Work out the finished part from the listing and answer in its coordinate system (mm). A direction names the side the tool comes from. Round coordinates to 2 decimals unless told otherwise and drop trailing zeros. Order: outer loops, then holes, each group sorted by start corner. A loop starts at its lowest first (then second) coordinate and runs counter-clockwise, first axis right, second up. Notation, with made-up numbers: (-15, 89.5) - (-8, 89.5) arc R34 cw to (-8, 125.5) - close; hole circle Ø4 at (-11, 54). An arc over 180 degrees is marked (long way). Answer in a Markdown table with one row per item.
from build123d import *

# Parameters (mm, degrees)
SCHIZZO1_R                   = 7.5
SCHIZZO1_R_2                 = 2
ESTRUSIONE_ESTRUSIONE1_DEPTH = 4


with BuildPart() as part:
    # Schizzo1 → Estrusione-Estrusione1 (new body)
    with BuildSketch(Plane.XY):
        Polygon((0, 90), (0, 0), (35, 0), (35, -4), (45, -4), (45, 0), (135, 0), (135, -4), (145, -4), (145, 0), (235, 0), (235, -4), (245, -4), (245, 0), (335, 0), (335, -4), (345, -4), (345, 0), (435, 0), (435, -4), (445, -4), (445, 0), (490, 0), (490, 90), (445, 90), (445, 94), (435, 94), (435, 90), (345, 90), (345, 94), (335, 94), (335, 90), (245, 90), (245, 94), (235, 94), (235, 90), (145, 90), (145, 94), (135, 94), (135, 90), (45, 90), (45, 94), (35, 94), (35, 90), align=None)
        with Locations((457.5, 45)):
            Circle(SCHIZZO1_R, mode=Mode.SUBTRACT)
        with Locations((437.5, 45)):
            Circle(SCHIZZO1_R_2, mode=Mode.SUBTRACT)
        with Locations((467.5, 27.679491924)):
            Circle(SCHIZZO1_R_2, mode=Mode.SUBTRACT)
        with Locations((467.5, 62.320508076)):
            Circle(SCHIZZO1_R_2, mode=Mode.SUBTRACT)
        Polygon((50, 77.928932188), (50, 12.071067812), (82.928932188, 45), align=None, mode=Mode.SUBTRACT)
        Polygon((130, 77.928932188), (130, 12.071067812), (97.071067812, 45), align=None, mode=Mode.SUBTRACT)
        Polygon((57.071067812, 85), (90, 52.071067812), (122.928932188, 85), align=None, mode=Mode.SUBTRACT)
        Polygon((123.1448388, 4.784093388), (57.077189669, 5.006121857), (90, 37.928932188), align=None, mode=Mode.SUBTRACT)
        Polygon((150, 77.928932188), (150, 12.071067812), (182.928932188, 45), align=None, mode=Mode.SUBTRACT)
        Polygon((230, 77.928932188), (230, 12.071067812), (197.071067812, 45), align=None, mode=Mode.SUBTRACT)
        Polygon((157.071067812, 85), (190, 52.071067812), (222.928932188, 85), align=None, mode=Mode.SUBTRACT)
        Polygon((223.1448388, 4.784093388), (157.077189669, 5.006121857), (190, 37.928932188), align=None, mode=Mode.SUBTRACT)
        Polygon((250, 77.928932188), (250, 12.071067812), (282.928932188, 45), align=None, mode=Mode.SUBTRACT)
        Polygon((330, 77.928932188), (330, 12.071067812), (297.071067812, 45), align=None, mode=Mode.SUBTRACT)
        Polygon((257.071067812, 85), (290, 52.071067812), (322.928932188, 85), align=None, mode=Mode.SUBTRACT)
        Polygon((323.1448388, 4.784093388), (257.077189669, 5.006121857), (290, 37.928932188), align=None, mode=Mode.SUBTRACT)
        Polygon((350, 77.928932188), (350, 12.071067812), (382.928932188, 45), align=None, mode=Mode.SUBTRACT)
        Polygon((430, 77.928932188), (430, 12.071067812), (397.071067812, 45), align=None, mode=Mode.SUBTRACT)
        Polygon((357.071067812, 85), (390, 52.071067812), (422.928932188, 85), align=None, mode=Mode.SUBTRACT)
        Polygon((423.1448388, 4.784093388), (357.077189669, 5.006121857), (390, 37.928932188), align=None, mode=Mode.SUBTRACT)
    extrude(amount=ESTRUSIONE_ESTRUSIONE1_DEPTH)


solid = part.part
1) Find section A-A, the plane x = 457.5. Give the vertices of the cut face in (y, z), then the cut area to 3 significant figures.
Filled in:
| item | result |
|---|---|
| outline | (0, 0) - (37.5, 0) - (37.5, 4) - (0, 4) - close; (52.5, 0) - (90, 0) - (90, 4) - (52.5, 4) - close |
| area | 300 mm^2 |
2) Find section B-B, the plane y = 69.5. Give the number of separate pieces and of enclosed holes in the cut face, then the cut area to 3 significant figures.
Filled in:
| item | result |
|---|---|
| separate pieces | 13 |
| enclosed holes | 0 |
| area | 1,130 mm^2 |
3) The mould has two halves that part along Y. Classify faces 3 (the face through (242, 46, 4)), 4 (the face through (366.695, 61.234, 1.972)): released by +Y, released by -Y, zero draft, split by the parting line, or undercut.
Filled in:
| item | result |
|---|---|
| face 3 | zero draft |
| face 4 | undercut |
4) Which of the six approach directions +Z, -Z, +X, -X, +Y, -Y give full straight-line access (tool end or side, diameter ignored) to faces 1 (the face through (242, 46, 0)), 2 (the face through (266.234, 28.305, 1.972))?
Filled in:
| item | result |
|---|---|
| face 1 | -Z, +X, -X, +Y, -Y |
| face 2 | +Z, -Z |
5) Find the intervals of material crossed by probe 1 along Y at (x, z) = (467.5, 1.75); probe 2 along Y at (x, z) = (102.5, 1.4); probe 3 along Y at (x, z) = (457.5, 1.25), in increasing order. Write a range as from..to.
Filled in:
| item | result |
|---|---|
| probe 1 | y = 0..25.68, 29.68..60.32, 64.32..90 |
| probe 2 | y = 0..4.85, 25.43..39.57, 50.43..64.57, 85..90 |
| probe 3 | y = 0..37.5, 52.5..90 |
6) Each of these flat-tipped pins is pushed along its axis until it touches: pin 1 (1.2 mm diameter, centred on y = 93, z = 1.5, fed in from -X); pin 2 (2 mm diameter, centred on y = 45, z = 2.5, fed in from -X); pin 3 (1.2 mm diameter, centred on x = 380.5, z = 1.5, fed in from -Y); pin 4 (1.2 mm diameter, centred on x = 311, z = 1, fed in from +Y). Where does it stop, or does it pass through?
Filled in:
| item | result |
|---|---|
| pin 1 | stops at x = 35 |
| pin 2 | stops at x = 0 |
| pin 3 | stops at y = 0 |
| pin 4 | stops at y = 90 |
